The figure shows three views and two pictorial views of one solid part (mm, origin at its lowest corner). Answer the questions. A direction names the side the tool comes from. Give positions to 0.01 mm unless a question says otherwise; leave off trailing zeros. Write each loop counter-clockwise with the first axis right and the second up, starting at its lowest first coordinate (ties: lowest second). Pieces come first, ordered by that corner, then holes. Notation, with made-up numbers: M -20.5,28.5 L 3.5,28.5 A19 cw 3.5,40.5 Z; hole C -14,14.5 d5. An arc over 180 degrees is marked long. Return JSON: item names as keys, results as strings.
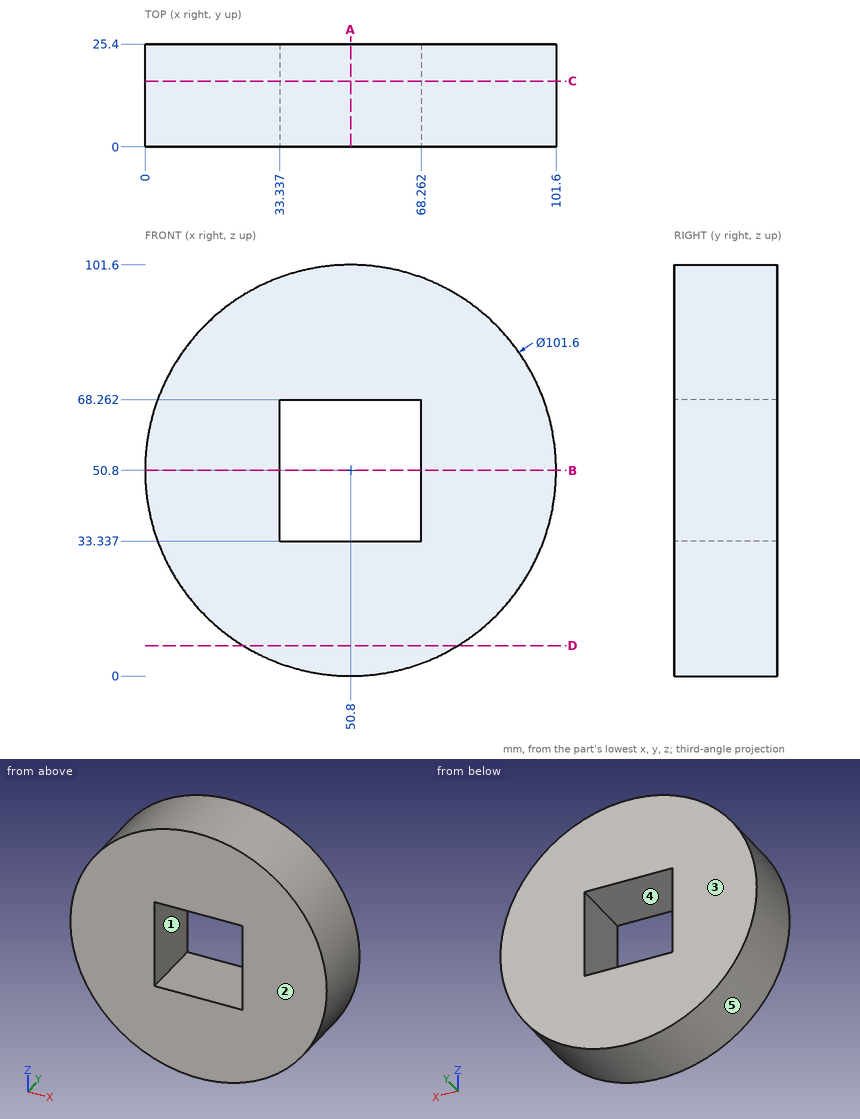
Item 1: A cutting plane is placed at B-B, the plane z = 50.8. Write down the section's boundary in (x, y), plus the area to 3 significant figures.
Geometry results:
{"outline": "M 0,0 L 33.34,0 L 33.34,25.4 L 0,25.4 Z; M 68.26,0 L 101.6,0 L 101.6,25.4 L 68.26,25.4 Z", "area": "1,690 mm2"}
Item 2: Given pin 1 Ø6 at (x, y) = (15.5, 15.5) entering from -Z; pin 2 Ø7.5 at (x, y) = (49.5, 16) entering from -Z; pin 3 Ø1 at (x, y) = (23, 8) entering from -Z, each flat-ended and moving along its own axis, determine where each tip first touches the part or whether it passes through.
Geometry results:
{"pin 1": "stops at z = 11.59", "pin 2": "stops at z = 0", "pin 3": "stops at z = 7.96"}
Item 3: A cutting plane is placed at C-C, the plane y = 16.25. Write down the section's boundary in (x, z).
Geometry results:
{"outline": "C 50.8,50.8 d101.6; hole M 33.34,33.34 L 68.26,33.34 L 68.26,68.26 L 33.34,68.26 Z"}
Item 4: A cutting plane is placed at A-A, the plane x = 50.8. Write down the section's boundary in (y, z), plus the area to 3 significant figures.
Geometry results:
{"outline": "M 0,0 L 25.4,0 L 25.4,33.34 L 0,33.34 Z; M 0,68.26 L 25.4,68.26 L 25.4,101.6 L 0,101.6 Z", "area": "1,690 mm2"}
Item 5: Determine the mould class of the marked faces 3, 4 and 5 for opening direction Z: +Z half, -Z half, draft (parallel to the pull), parting line (faces both ways), or undercut.
Geometry results:
{"face 3": "draft", "face 4": "undercut", "face 5": "parting line"}
Item 6: Which of the six approach directions +Z, -Z, +X, -X, +Y, -Y give full straight-line access (tool end or side, diameter ignored) to the marked faces 1 and 2?
Geometry results:
{"face 1": "+Y, -Y", "face 2": "+Z, -Z, +X, -X, -Y"}
Item 7: A cutting plane is placed at D-D, the plane z = 7.5. Write down the section's boundary in (x, y) (1 decimal).
Geometry results:
{"outline": "M 24.2,0 L 77.4,0 L 77.4,25.4 L 24.2,25.4 Z"}
Item 8: Find the intervals of material crossed by line 1 (Z direction, x = 59, y = 17) (1 decimal); line 2 (X direction, y = 7.75, z = 42); line 3 (X direction, y = 16.25, z = 36.5) (1 decimal), in increasing order.
Geometry results:
{"line 1": "z = 0.7 to 33.3, 68.3 to 100.9", "line 2": "x = 0.77 to 33.34, 68.26 to 100.83", "line 3": "x = 2.1 to 33.3, 68.3 to 99.5"}
